Build history of the part. All positions in model axes, mm. Round coordinates to 2 decimals unless told otherwise and drop trailing zeros. Loops run counter-clockwise (first coordinate to the right, second up) from the corner with the lowest first, then second, coordinate; pieces in that order, holes last. Notation, with made-up numbers: (-34.5, -11.75) - (-25.5, -11.75) arc R23 cw to (-25.5, 4.25) - close; hole circle Ø7 at (10.25, 6). An arc over 180 degrees is marked (long way). Use one line per item in the form item = value. Start each with the question number.
Q1. Saw through at B-B (y = 17.5). Give the cut face in (x, z), then the cut area to 3 significant figures.
Q2. Saw through at A-A (x = -42). Give the cut face in (y, z), then the cut area to 3 significant figures.
Q3. Drill centre lines: line 1 (X direction, y = -0.5, z = 2.1); line 2 (Y direction, x = -30.5, z = 2.7); line 3 (Y direction, x = -17, z = 0.45). Where is each one in solid material? Low to high.
Q4. Saw through at C-C (z = 2.8). Give the cut face in (x, y), then the cut area to 3 significant figures.
Q5. Pin check, flat tips, straight feed: pin 1 (1.5 mm diameter, centred on y = -32.5, z = 2.5, fed in from +X); pin 2 (1.6 mm diameter, centred on y = -14.5, z = 3.5, fed in from -X); pin 3 (0.6 mm diameter, centred on x = 39.5, z = 2.5, fed in from -Y). Stop position of each tip, or through.
```python
from build123d import *

# Parameters (mm, degrees)
SKETCH1_W           = 199
SKETCH1_H           = 107
BOSS_EXTRUDE1_DEPTH = 2
SKETCH2_W           = 193
SKETCH2_H           = 90
BOSS_EXTRUDE2_DEPTH = 2.5
FILLET2_R           = 0.5
FILLET3_R           = 0.5


with BuildPart() as part:
    # Sketch1 → Boss-Extrude1 (new body)
    with BuildSketch(Plane.XY):
        Rectangle(SKETCH1_W, SKETCH1_H)
    extrude(amount=BOSS_EXTRUDE1_DEPTH)

    # Sketch2 → Boss-Extrude2 (add)
    with BuildSketch(Plane.XY.offset(2)):
        with Locations((0, 1.5)):
            Rectangle(SKETCH2_W, SKETCH2_H)
    extrude(amount=BOSS_EXTRUDE2_DEPTH)

    # Fillet2
    fillet2_edges = [part.edges().sort_by_distance(p)[0] for p in [
        (-96.5, 1.5, 4.5),
        (0, -43.5, 4.5),
        (96.5, 1.5, 4.5),
        (0, 46.5, 4.5),
    ]]
    fillet(fillet2_edges, radius=FILLET2_R)

    # Fillet3
    fillet3_edges = [part.edges().sort_by_distance(p)[0] for p in [
        (0, -53.5, 0),
        (-99.5, 0, 0),
        (0, 53.5, 0),
        (99.5, 0, 0),
    ]]
    fillet(fillet3_edges, radius=FILLET3_R)


solid = part.part
```
Report:
q1.outline = (-99.5, 0.5) arc R0.5 ccw to (-99, 0) - (99, 0) arc R0.5 ccw to (99.5, 0.5) - (99.5, 2) - (96.5, 2) - (96.5, 4) arc R0.5 ccw to (96, 4.5) - (-96, 4.5) arc R0.5 ccw to (-96.5, 4) - (-96.5, 2) - (-99.5, 2) - close
q1.area = 880 mm²
q2.outline = (-53.5, 0.5) arc R0.5 ccw to (-53, 0) - (53, 0) arc R0.5 ccw to (53.5, 0.5) - (53.5, 2) - (46.5, 2) - (46.5, 4) arc R0.5 ccw to (46, 4.5) - (-43, 4.5) arc R0.5 ccw to (-43.5, 4) - (-43.5, 2) - (-53.5, 2) - close
q2.area = 439 mm²
q3.line_1 = -96.5 to 96.5
q3.line_2 = -43.5 to 46.5
q3.line_3 = -53.5 to 53.5
q4.outline = (-96.5, -43.5) - (96.5, -43.5) - (96.5, 46.5) - (-96.5, 46.5) - close
q4.area = 17,400 mm²
q5.pin_1 = 99.5
q5.pin_2 = -96.5
q5.pin_3 = -43.5
